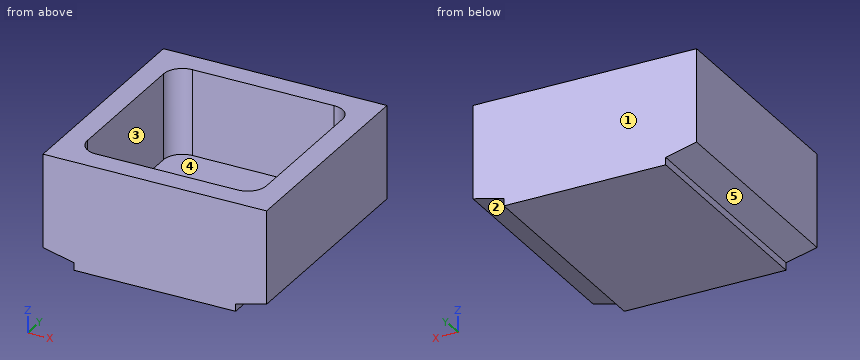
```python
from build123d import *

# Parameters (mm, degrees)
F0_W     = 76.2
F0_H     = 76.2
F1_DEPTH = 36.83
F3_DEPTH = 76.201
F5_DEPTH = 29.21
F6_SCALE = 0.6666


with BuildPart() as f1:
    # F0 (on Top) → F1 (new body)
    with BuildSketch(Plane.XY):
        Rectangle(F0_W, F0_H)
    extrude(amount=-F1_DEPTH)

    # F2 (on face) → F3 (cut, through all)
    with BuildSketch(Plane.XZ.offset(38.1)):
        Polygon((27.559, -34.29), (27.559, -36.83), (38.1, -36.83), (38.1, -31.75), align=None)
        Polygon((-38.1, -36.83), (-27.559, -36.83), (-27.559, -34.29), (-38.1, -31.75), align=None)
    extrude(amount=-F3_DEPTH, mode=Mode.SUBTRACT)

    # F4 (on face) → F5 (cut)
    with BuildSketch(Plane.XY):
        with BuildLine():
            ThreePointArc((30.48, 24.13), (28.6201280605, 28.6201280605), (24.13, 30.48))
            Line((24.13, 30.48), (-24.13, 30.48))
            ThreePointArc((-24.13, 30.48), (-28.6201280605, 28.6201280605), (-30.48, 24.13))
            Line((-30.48, 24.13), (-30.48, -24.13))
            ThreePointArc((-30.48, -24.13), (-28.6201280605, -28.6201280605), (-24.13, -30.48))
            Line((-24.13, -30.48), (24.13, -30.48))
            ThreePointArc((24.13, -30.48), (28.6201280605, -28.6201280605), (30.48, -24.13))
            Line((30.48, -24.13), (30.48, 24.13))
        make_face()
    extrude(amount=-F5_DEPTH, mode=Mode.SUBTRACT)


with BuildPart() as f1_1:
    # F6: moved
    add(f1.part.scale(F6_SCALE))


solid = f1_1.part
```
The listing builds one solid part. Answer for the finished solid, in the listing's coordinates (mm). Face numbers are marked on the shaded views. A direction names the side the tool comes from. Give positions to 0.01 mm unless a question says otherwise; leave off trailing zeros. Loops run counter-clockwise (first coordinate to the right, second up) from the corner with the lowest first, then second, coordinate; pieces in that order, holes last. Notation, with made-up numbers: (21.5, 23.5) - (57.5, 23.5) arc R31 cw to (57.5, 57.5) - close; hole circle Ø7 at (46.25, 71). An arc over 180 degrees is marked (long way). Return JSON: item names as keys, results as strings. Group by question number.
1. Find section D-D (y = 22). Write down the section's boundary in (x, z).
2. Given pin 1 Ø20.5 at (x, y) = (5, -3.5) entering from +Z; pin 2 Ø0.8 at (y, z) = (4, -24) entering from -X; pin 3 Ø0.5 at (y, z) = (6, -23.5) entering from +X, each flat-ended and moving along its own axis, determine where each tip first touches the part or whether it passes through.
3. Straight lines are drawn through the part: line 1 (X direction, y = -7, z = -7.5); line 2 (Z direction, x = 13, y = 3). For each, find the intervals that lie inside material, in ascending order. Write a range as [from, to].
4. Find section A-A (z = -10). Write down the section's boundary in (x, y).
5. Find section C-C (x = -15). Write down the section's boundary in (y, z), then the cut area to 3 significant figures.
6. Determine the mould class of the marked faces 1, 2 and 3 for opening direction X: pulls with the +X half, pulls with the -X half, needs draft (parallel to the pull), parting line crosses it, or undercut.
7. Find section B-B (y = 6). Write down the section's boundary in (x, z).
8. Which of the six approach directions +Z, -Z, +X, -X, +Y, -Y give full straight-line access (tool end or side, diameter ignored) to the marked faces 4 and 5?
Verdict:
{
 "1": {"outline": "(-25.4, -21.16) - (-18.37, -22.86) - (-18.37, -24.55) - (18.37, -24.55) - (18.37, -22.86) - (25.4, -21.16) - (25.4, 0) - (-25.4, 0) - close"},
 "2": {"pin 1": "stops at z = -19.47", "pin 2": "stops at x = -18.37", "pin 3": "stops at x = 18.37"},
 "3": {"line 1": "x = [-25.4, -20.32], [20.32, 25.4]", "line 2": "z = [-24.55, -19.47]"},
 "4": {"outline": "(-25.4, -25.4) - (25.4, -25.4) - (25.4, 25.4) - (-25.4, 25.4) - close; hole (-20.32, -16.09) arc R4.23 ccw to (-16.09, -20.32) - (16.09, -20.32) arc R4.23 ccw to (20.32, -16.09) - (20.32, 16.09) arc R4.23 ccw to (16.09, 20.32) - (-16.09, 20.32) arc R4.23 ccw to (-20.32, 16.09) - close"},
 "5": {"outline": "(-25.4, -24.55) - (25.4, -24.55) - (25.4, 0) - (20.32, 0) - (20.32, -19.47) - (-20.32, -19.47) - (-20.32, 0) - (-25.4, 0) - close", "area": "456 mm^2"},
 "6": {"face 1": "needs draft", "face 2": "pulls with the +X half", "face 3": "undercut"},
 "7": {"outline": "(-25.4, -21.16) - (-18.37, -22.86) - (-18.37, -24.55) - (18.37, -24.55) - (18.37, -22.86) - (25.4, -21.16) - (25.4, 0) - (20.32, 0) - (20.32, -19.47) - (-20.32, -19.47) - (-20.32, 0) - (-25.4, 0) - close"},
 "8": {"face 4": "+Z", "face 5": "-Z, -X, +Y, -Y"}
}
